Design review of the part built by this model. Coordinates are the model's own, in mm. Round coordinates to 2 decimals unless told otherwise and drop trailing zeros. Order: outer loops, then holes, each group sorted by start corner. A loop starts at its lowest first (then second) coordinate and runs counter-clockwise, first axis right, second up. Notation, with made-up numbers: (-6.5, 35.25) - (33.5, 35.25) arc R6 ccw to (33.5, 43.25) - close; hole circle Ø9 at (-11.5, -16). An arc over 180 degrees is marked (long way). Use CSV: the item, a comma, the result in double quotes.
Autodesk Inventor part; units mm, degrees
ref_plane "YZ Plane" through (0, 0, 0) normal (1, 0, 0) x (0, 1, 0)
ref_plane "XZ Plane" through (0, 0, 0) normal (0, 1, 0) x (-1, 0, 0)
ref_plane "XY Plane" through (0, 0, 0) normal (0, 0, 1) x (1, 0, 0)
sketch "Sketch1" plane through (0, 0, 0) normal (0, 1, 0) x (-1, 0, 0)
  point P0 (0, 0)
sketch "Sketch2" plane through (0, 0, 0) normal (0, 1, 0) x (-1, 0, 0)
  line L0 (0, 0) -> (45.5, 0)
  line L1 (45.5, 0) -> (45.5, -35)
  line L2 (45.5, -35) -> (0, -35)
  line L3 (0, -35) -> (0, 0)
  dimension "d0" = 45.5
  dimension "d1" = 35
extrude "Extrusion1" add sketch "Sketch2" along normal blind 3
sketch "Sketch3" plane through (0, 3, 0) normal (0, 1, 0) x (1, 0, 0)
  circle A0 centre (-6, 6) radius 1
  line L0 (-45.5, 0) -> (0, 0)
  line L1 (0, 0) -> (0, 35)
  circle A1 centre (-6, 29) radius 1
  line L2 (0, 35) -> (-45.5, 35)
  dimension "d4" = 2
  dimension "d5" = 6
  dimension "d6" = 6
  dimension "d7" = 2
  dimension "d8" = 6
  dimension "d9" = 6
hole "Hole1" at (-6, 3, -6) at (-6, 3, -29) direction (0, -1, 0) diameter 3 end through all
properties part number "FrontSupport" material "Wood (Birch)"
1) We need section C-C (z = -28). Give the boundary of the cut face in (x, y), then the cut area to 3 significant figures.
Data:
outline,"(-45.5, 0) - (-7.12, 0) - (-7.12, 3) - (-45.5, 3) - close; (-4.88, 0) - (0, 0) - (0, 3) - (-4.88, 3) - close"
area,"130 mm2"
2) We need section A-A (x = -6). Give the boundary of the cut face in (y, z), then the cut area to 3 significant figures.
Data:
outline,"(0, -35) - (3, -35) - (3, -30.5) - (0, -30.5) - close; (0, -27.5) - (3, -27.5) - (3, -7.5) - (0, -7.5) - close; (0, -4.5) - (3, -4.5) - (3, 0) - (0, 0) - close"
area,"87.0 mm2"
3) We need section B-B (z = -6). Give the boundary of the cut face in (x, y).
Data:
outline,"(-45.5, 0) - (-7.5, 0) - (-7.5, 3) - (-45.5, 3) - close; (-4.5, 0) - (0, 0) - (0, 3) - (-4.5, 3) - close"
4) To check wall thickness, follow L1, parallel to Z at x = -6, y = 1.45; L2, parallel to X at y = 0.85, z = -6. State the ranges of each line that lie inside material, in increasing order. Write a range as from..to.
Data:
L1,"z = -35..-30.5, -27.5..-7.5, -4.5..0"
L2,"x = -45.5..-7.5, -4.5..0"
5) Insertion check: pin 1 Ø5 at (x, z) = (-28, -31) entering from -Y. The pin has a flat end and moves straight along its axis. Give the tip position at first contact, or say it passes through.
Data:
pin 1,"stops at y = 0"
